Check sheet for the modelled part. Datum: model origin and axes. Units: mm. A direction names the side the tool comes from. Coordinates: 2 decimals unless noted, no trailing zeros. Loops run counter-clockwise (first coordinate to the right, second up) from the corner with the lowest first, then second, coordinate; pieces in that order, holes last. Notation, with made-up numbers: (44.25, 82.5) - (69.25, 82.5) arc R21 ccw to (69.25, 90.5) - close; hole circle Ø9 at (-12.75, 11.5). An arc over 180 degrees is marked (long way). Write each question's results on one line, items separated by ' | '. Start each with the question number.
1. Cross-section at A-A (x = 212). Record the cut outline in (y, z).
2. Cross-section at B-B (y = 0). Give the number of separate pieces and of enclosed holes in the cut face, and give its area (3 significant figures).
3. Gauge pin test, flat ends, axial feed: P1, Ø6, axis at x = 130, y = 0.5, coming from the +Z side; P2, Ø2.5, axis at y = 5, z = 2.5, coming from the +X side; P3, Ø1.5, axis at x = 198, y = -1, coming from the -Z side. Record the tip position at first contact, or that the pin passes through.
4. Cross-section at D-D (x = 31.5). Record the cut outline in (y, z).
5. Draft check along Z on faces 3 (the face through (3, 0, 5.5)), 4 (the face through (3, 0, -0.5)), 5 (the face through (133, 0, 0)), 6 (the face through (-10, 0, -3)). Enter one of: released by +Z, released by -Z, zero draft, split by the parting line, or undercut.
6. Tool access check on faces 1 (the face through (133, 0, 5)), 2 (the face through (7, 0, -5)). Record the directions out of +Z, -Z, +X, -X, +Y, -Y that give a thin tool (end or side, any length) a straight path to the whole face; none if there is none.
7. Cross-section at C-C (x = 75). Record the cut outline in (y, z), and give its area (3 significant figures).
8. Thickness scan on line 1 (Y direction, x = 215.5, z = 2.5); line 2 (Y direction, x = 0, z = -2); line 3 (Z direction, x = 53, y = 4.5). Record the ranges inside material, lowest first. Write a range as [from, to].
```python
from build123d import *

# Parameters (mm, degrees)
SKETCH1_R                = 2
BOSS_EXTRUDE1_DEPTH      = 5
BOSS_EXTRUDE2_DEPTH      = 5
BOSS_EXTRUDE2_DEPTH_BACK = 10
SKETCH2_R                = 2
SKETCH4_W                = 40
SKETCH4_H                = 6
CUT_EXTRUDE1_DEPTH       = 232.084400166
FILLET1_R                = 10
FILLET2_R                = 3
SKETCH5_R                = 1.6
CUT_EXTRUDE2_DEPTH       = 20


# Some blends are built 0.0001 mm under size
with BuildPart() as part:
    # Sketch1 → Boss-Extrude1 (new body)
    with BuildSketch(Plane.XY):
        with BuildLine():
            Line((0, 10), (230, 10))
            Line((230, 10), (230, -10))
            Line((230, -10), (0, -10))
            ThreePointArc((0, -10), (-10, 0), (0, 10))
        make_face()
        Circle(SKETCH1_R, mode=Mode.SUBTRACT)
    extrude(amount=BOSS_EXTRUDE1_DEPTH)

    # Sketch2 → Boss-Extrude2 (add, two sides: drawn at the far end of the back side and taken through both)
    with BuildSketch(Plane.XY.offset(5).offset(-BOSS_EXTRUDE2_DEPTH_BACK)):
        with BuildLine():
            Line((25, -10), (25, 10))
            Line((25, 10), (0, 10))
            ThreePointArc((0, 10), (-10, 0), (0, -10))
            Line((0, -10), (25, -10))
        make_face()
        Circle(SKETCH2_R, mode=Mode.SUBTRACT)
    extrude(amount=BOSS_EXTRUDE2_DEPTH + BOSS_EXTRUDE2_DEPTH_BACK)

    # Sketch4 → Cut-Extrude1 (cut, through all)
    with BuildSketch(Plane(origin=(0, 10, 0), x_dir=(1, 0, 0), z_dir=(0, 1, 0))):
        with Locations((0, -2.5)):
            Rectangle(SKETCH4_W, SKETCH4_H)
    extrude(amount=-CUT_EXTRUDE1_DEPTH, mode=Mode.SUBTRACT)

    # Fillet1
    # the kernel refuses this fillet: 10 mm, written as the material it adds along each edge
    with BuildSketch(Plane(origin=(25, -10, 5), x_dir=(1, 0, 0), z_dir=(0, 1, 0))) as fillet1_piece_1:
        with BuildLine():
            CenterArc((8.660254038, -10), FILLET1_R, 90, 60)
            Line((0, -5), (-0.173205081, -4.9))
            ThreePointArc((-0.173205081, -4.9), (-0.2, -2.5), (-0.2, 0))
            Line((-0.2, 0), (0, 0.2))
            Line((0, 0.2), (8.660254038, 0.2))
            Line((8.660254038, 0.2), (8.660254038, 0))
        make_face()
    extrude(amount=20)
    with BuildSketch(Plane(origin=(25, -10, 0), x_dir=(0, 0, -1), z_dir=(0, 1, 0))) as fillet1_piece_2:
        with BuildLine():
            CenterArc((10, -8.660254038), FILLET1_R, 120, 60)
            Line((0, -8.660254038), (-0.2, -8.660254038))
            Line((-0.2, -8.660254038), (-0.2, 0))
            Line((-0.2, 0), (0, 0.2))
            ThreePointArc((0, 0.2), (2.5, 0.2), (4.9, 0.173205081))
            Line((4.9, 0.173205081), (5, 0))
        make_face()
    extrude(amount=20)

    # Fillet2
    fillet2_edges = [part.edges().sort_by_distance(p)[0] for p in [
        (20, 0, -0.5),
        (20, 0, 5.5),
    ]]
    fillet(fillet2_edges, radius=FILLET2_R - 0.0001)  # a hair under: the kernel refuses the full size

    # Sketch5 → Cut-Extrude2 (cut)
    with BuildSketch(Plane(origin=(230, 0, 0), x_dir=(0, 0, -1), z_dir=(1, 0, 0))):
        with Locations((-2.5, 5)):
            Circle(SKETCH5_R)
    extrude(amount=-CUT_EXTRUDE2_DEPTH, mode=Mode.SUBTRACT)


solid = part.part
```
Established:
1) outline: (-10, 0) - (10, 0) - (10, 5) - (-10, 5) - close; hole circle Ø3.2 at (5, 2.5)
2) separate pieces: 3 | enclosed holes: 0 | area: 1,360 mm^2
3) P1: z = 5 | P2: x = 210 | P3: z = 0
4) outline: (-10, -0.24) - (10, -0.24) - (10, 5.24) - (-10, 5.24) - close
5) face 3: undercut | face 4: undercut | face 5: released by -Z | face 6: zero draft
6) face 1: +Z, +X, +Y, -Y | face 2: -Z, +X, -X, +Y, -Y
7) outline: (-10, 0) - (10, 0) - (10, 5) - (-10, 5) - close | area: 100 mm^2
8) line 1: [-10, 3.4], [6.6, 10] | line 2: [-10, -2], [2, 10] | line 3: [0, 5]
